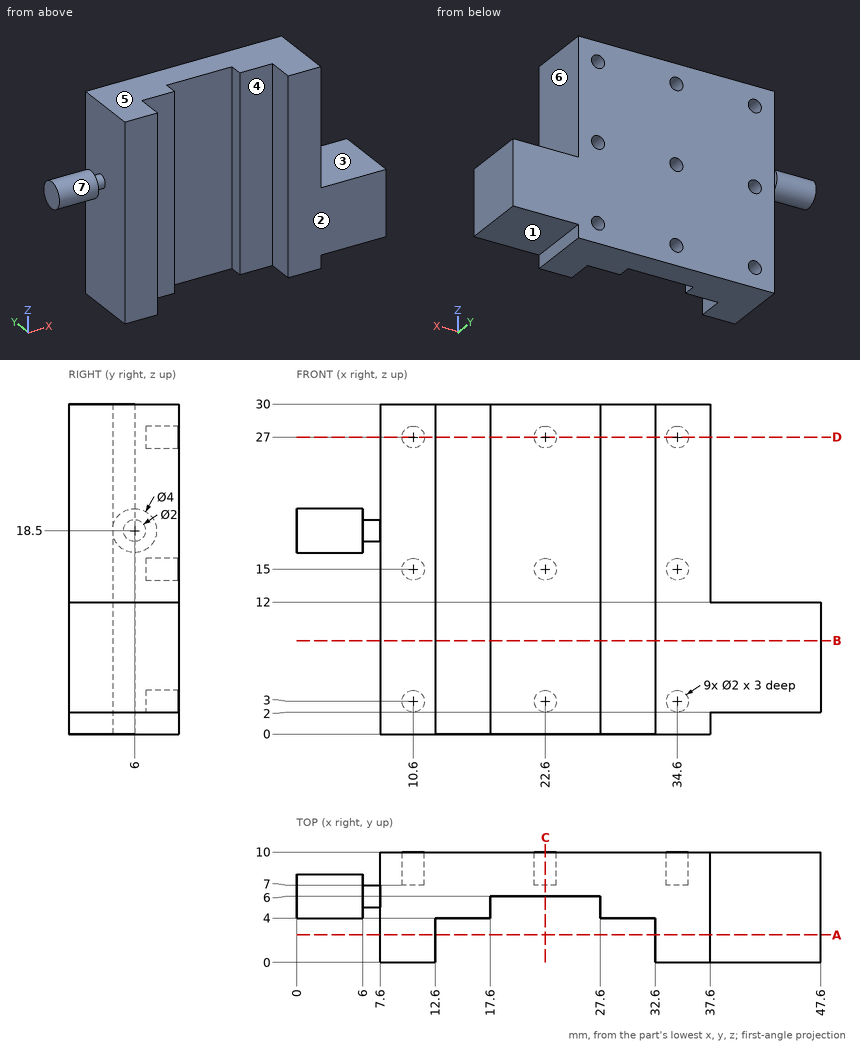
Study the drawing (mm; zero at the part's minimum x, y, z) and answer. A direction names the side the tool comes from. Give positions to 0.01 mm unless a question says otherwise; leave off trailing zeros. Write each loop counter-clockwise with the first axis right and the second up, starting at its lowest first coordinate (ties: lowest second). Pieces come first, ordered by that corner, then holes. Notation, with made-up numbers: M 42.25,8.5 L 97.25,8.5 A14 cw 97.25,32.5 Z; hole C -4,21 d5. An arc over 180 degrees is marked long. Put each result on its own line as item: value. Start each with the question number.
1. The part is cut by section A-A, the plane y = 2.5. Give the vertices of the cut face in (x, z), and give its area (3 significant figures).
2. Each of these flat-tipped pins is pushed along its axis until it touches: pin 1 Ø2 at (x, z) = (29, 7.5) entering from -Y; pin 2 Ø4 at (y, z) = (8, 24) entering from -X; pin 3 Ø1.6 at (x, z) = (34.5, 27) entering from +Y. Where does it stop, or does it pass through?
3. For a pull along Z with two mould halves and no side action, classify the marked faces 5, 6 and 7 as released by +Z, released by -Z, zero draft, split by the parting line, or undercut.
4. Consider line 1 along X through (y, z) = (8, 27); line 2 along X through (y, z) = (8.4, 3); line 3 along X through (y, z) = (1, 7.5). Determine where each line is inside the solid, lowest interval first.
5. The part is cut by section B-B, the plane z = 8.5. Give the vertices of the cut face in (x, y), and give its area (3 significant figures).
6. The part is cut by section D-D, the plane z = 27. Give the vertices of the cut face in (x, y), and give its area (3 significant figures).
7. The part is cut by section C-C, the plane x = 22.6. Give the vertices of the cut face in (y, z), and give its area (3 significant figures).
8. Which of the six approach directions +Z, -Z, +X, -X, +Y, -Y give full straight-line access (tool end or side, diameter ignored) to the marked faces 1, 2, 3 and 4?
Final values:
1. outline: M 7.6,0 L 12.6,0 L 12.6,30 L 7.6,30 Z; M 32.6,0 L 37.6,0 L 37.6,2 L 47.6,2 L 47.6,12 L 37.6,12 L 37.6,30 L 32.6,30 Z
1. area: 400 mm²
2. pin 1: stops at y = 4
2. pin 2: stops at x = 7.6
2. pin 3: stops at y = 7
3. face 5: released by +Z
3. face 6: zero draft
3. face 7: split by the parting line
4. line 1: x = 7.6 to 9.6, 11.6 to 21.6, 23.6 to 33.6, 35.6 to 37.6
4. line 2: x = 7.6 to 9.6, 11.6 to 21.6, 23.6 to 33.6, 35.6 to 47.6
4. line 3: x = 7.6 to 12.6, 32.6 to 47.6
5. outline: M 7.6,0 L 12.6,0 L 12.6,4 L 17.6,4 L 17.6,6 L 27.6,6 L 27.6,4 L 32.6,4 L 32.6,0 L 47.6,0 L 47.6,10 L 7.6,10 Z
5. area: 300 mm²
6. outline: M 7.6,0 L 12.6,0 L 12.6,4 L 17.6,4 L 17.6,6 L 27.6,6 L 27.6,4 L 32.6,4 L 32.6,0 L 37.6,0 L 37.6,10 L 35.6,10 L 35.6,7 L 33.6,7 L 33.6,10 L 23.6,10 L 23.6,7 L 21.6,7 L 21.6,10 L 11.6,10 L 11.6,7 L 9.6,7 L 9.6,10 L 7.6,10 Z
6. area: 182 mm²
7. outline: M 6,0 L 10,0 L 10,2 L 7,2 L 7,4 L 10,4 L 10,14 L 7,14 L 7,16 L 10,16 L 10,26 L 7,26 L 7,28 L 10,28 L 10,30 L 6,30 Z
7. area: 102 mm²
8. face 1: -Z, +X, +Y, -Y
8. face 2: +Z, -Z, +X, -X, -Y
8. face 3: +Z, +X, +Y, -Y
8. face 4: +Z, -Z, -Y
